```python
from build123d import *

# Parameters (mm, degrees)
F1_DEPTH = 15
F0_R     = 2.5
F3_DEPTH = 2.5
F2_R     = 4
F4_DEPTH = 5.001
F5_R     = 5
F6_R     = 1
F7_R     = 5
F2_R_2   = 8
F8_DEPTH = 3


with BuildPart() as f1:
    # F0 (on Front) → F1 (new body, symmetric)
    with BuildSketch(Plane.XZ):
        Polygon((-35.0252258055, 0), (0, 0), (35.0252258055, 0), (62.5, -10), (92.5, -10), (92.5, -5), (78.5, -5), (63.3816349035, -5), (35.906860709, 5), (0, 5), (-35.906860709, 5), (-63.3816349035, -5), (-78.5, -5), (-92.5, -5), (-92.5, -10), (-62.5, -10), align=None)
    extrude(amount=F1_DEPTH, both=True)

    # F0 (on Front) → F3 (join, symmetric)
    with BuildSketch(Plane.XZ):
        Polygon((-35.0252258055, 0), (0, 0), (35.0252258055, 0), (62.5, -10), (92.5, -10), (92.5, -5), (78.5, -5), (63.3816349035, -5), (35.906860709, 5), (0, 5), (-35.906860709, 5), (-63.3816349035, -5), (-78.5, -5), (-92.5, -5), (-92.5, -10), (-62.5, -10), align=None)
        Polygon((-30, 30), (-78.5, -5), (-63.3816349035, -5), (-35.906860709, 5), (0, 5), (35.906860709, 5), (63.3816349035, -5), (78.5, -5), (30, 30), (0, 30), align=None)
        with Locations((-10, 20)):
            Circle(F0_R, mode=Mode.SUBTRACT)
        with Locations((10, 20)):
            Circle(F0_R, mode=Mode.SUBTRACT)
    extrude(amount=F3_DEPTH, both=True)

    # F2 (on face) → F4 (cut, through all)
    with BuildSketch(Plane.XY.offset(-5)):
        with Locations((-82.5, 0)):
            Circle(F2_R)
        with Locations((82.5, 0)):
            Circle(F2_R)
    extrude(amount=-F4_DEPTH, mode=Mode.SUBTRACT)

    # F5
    f5_edges = [f1.edges().sort_by_distance(p)[0] for p in [
        (-63.381635, -8.75, -5),
        (-63.381635, 8.75, -5),
        (-35.906861, -8.75, 5),
        (-35.906861, 8.75, 5),
        (63.381635, 8.75, -5),
        (63.381635, -8.75, -5),
        (35.906861, -8.75, 5),
        (35.906861, 8.75, 5),
    ]]
    fillet(f5_edges, radius=F5_R)

    # F6
    f6_edges = [f1.edges().sort_by_distance(p)[0] for p in [
        (0, -2.5, 5),
        (0, 2.5, 5),
    ]]
    fillet(f6_edges, radius=F6_R)

    # F7
    f7_edges = [f1.edges().sort_by_distance(p)[0] for p in [
        (-92.5, -15, -7.5),
        (92.5, -15, -7.5),
        (92.5, 15, -7.5),
        (-92.5, 15, -7.5),
    ]]
    fillet(f7_edges, radius=F7_R)

    # F2 (on face) → F8 (join)
    with BuildSketch(Plane.XY.offset(-5)):
        with Locations((-82.5, 0)):
            Circle(F2_R_2)
        with Locations((-82.5, 0)):
            Circle(F2_R, mode=Mode.SUBTRACT)
        with Locations((82.5, 0)):
            Circle(F2_R_2)
        with Locations((82.5, 0)):
            Circle(F2_R, mode=Mode.SUBTRACT)
    extrude(amount=F8_DEPTH)


solid = f1.part
```
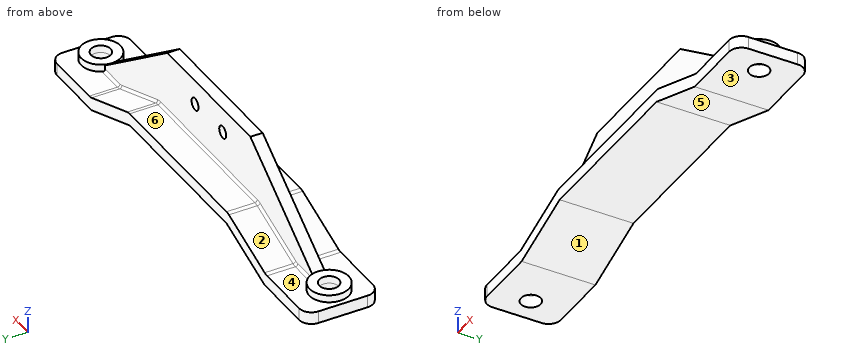
Could you check a few things on this model? Use its own coordinates, in mm. Face numbers are marked on the shaded views. A direction names the side the tool comes from. Coordinates: 2 decimals unless noted, no trailing zeros. Write each loop counter-clockwise with the first axis right and the second up, starting at its lowest first coordinate (ties: lowest second). Pieces come first, ordered by that corner, then holes. Notation, with made-up numbers: (-13, 20.5) - (7, 20.5) arc R14 ccw to (7, 32.5) - close; hole circle Ø5 at (54.25, 22.25). An arc over 180 degrees is marked (long way). Use a Markdown table: item, result.
Q1. Imagine slicing it at C-C (z = 20). List the corners of the cut face in (x, y) for me.
Geometry check:
| item | result |
|---|---|
| outline | (-43.86, -2.5) - (-12.5, -2.5) - (-12.5, 2.5) - (-43.86, 2.5) - close; (-7.5, -2.5) - (7.5, -2.5) - (7.5, 2.5) - (-7.5, 2.5) - close; (12.5, -2.5) - (43.86, -2.5) - (43.86, 2.5) - (12.5, 2.5) - close |
Q2. Thinking about a two-plate mould opening in X: for the marked faces 5 and 6, which applies, +X half, -X half, draft (parallel to the pull), parting line (faces both ways), or undercut?
Geometry check:
| item | result |
|---|---|
| face 5 | undercut |
| face 6 | draft |
Q3. Imagine slicing it at D-D (x = 4.5). List the corners of the cut face in (y, z) for me, and give its area (3 significant figures).
Geometry check:
| item | result |
|---|---|
| outline | (-15, 0) - (15, 0) - (15, 5) - (3.5, 5) arc R1 cw to (2.5, 6) - (2.5, 30) - (-2.5, 30) - (-2.5, 6) arc R1 cw to (-3.5, 5) - (-15, 5) - close |
| area | 275 mm2 |
Q4. Please list where these lines run through material, in increasing order: L1, parallel to Y at x = -82.5, z = -3.3; L2, parallel to Y at x = -82.5, z = -6.2; L3, parallel to Z at x = -10, y = 0.1.
Geometry check:
| item | result |
|---|---|
| L1 | y = -8 to -4, 4 to 8 |
| L2 | y = -15 to -4, 4 to 15 |
| L3 | z = 0 to 17.5, 22.5 to 30 |
Q5. Which directions (+Z, -Z, +X, -X, +Y, -Y) give clear straight access to the entire face, cutting with the end or side of a thin tool? Please do the marked faces 1, 2, 3 and 4.
Geometry check:
| item | result |
|---|---|
| face 1 | -Z, +Y, -Y |
| face 2 | +Z, +Y |
| face 3 | -Z, +X, -X, +Y, -Y |
| face 4 | +Z |
Q6. I'm going to push flat-ended pins straight in: pin 1 Ø13 at (x, y) = (-82.5, 0) entering from -Z; pin 2 Ø5 at (x, y) = (82.5, 3) entering from +Z; pin 3 Ø1 at (x, z) = (-6.5, 18) entering from -Y; pin 4 Ø8.5 at (x, y) = (-78, -2.5) entering from +Z. Where does each tip first touch, or does it pass through?
Geometry check:
| item | result |
|---|---|
| pin 1 | stops at z = -10 |
| pin 2 | stops at z = -2 |
| pin 3 | stops at y = -2.5 |
| pin 4 | stops at z = -1.57 |
Q7. Imagine slicing it at A-A (x = -82.5). List the corners of the cut face in (y, z) for me, and give its area (3 significant figures).
Geometry check:
| item | result |
|---|---|
| outline | (-15, -10) - (-4, -10) - (-4, -2) - (-8, -2) - (-8, -5) - (-15, -5) - close; (4, -10) - (15, -10) - (15, -5) - (8, -5) - (8, -2) - (4, -2) - close |
| area | 134 mm2 |
Q8. Imagine slicing it at B-B (y = 0). List the corners of the cut face in (x, z) for me.
Geometry check:
| item | result |
|---|---|
| outline | (-92.5, -10) - (-86.5, -10) - (-86.5, -2) - (-90.5, -2) - (-90.5, -5) - (-92.5, -5) - close; (-78.5, -10) - (-62.5, -10) - (-35.03, 0) - (35.03, 0) - (62.5, -10) - (78.5, -10) - (78.5, -2) - (74.5, -2) - (74.5, -2.11) - (30, 30) - (-30, 30) - (-74.5, -2.11) - (-74.5, -2) - (-78.5, -2) - close; (86.5, -10) - (92.5, -10) - (92.5, -5) - (90.5, -5) - (90.5, -2) - (86.5, -2) - close; hole circle Ø5 at (-10, 20); hole circle Ø5 at (10, 20) |
